Could you check a few things on this drawing? It's one solid part, dimensions in mm from its lowest x, y, z. Give positions to 0.01 mm unless a question says otherwise; leave off trailing zeros. Order: outer loops, then holes, each group sorted by start corner. A loop starts at its lowest first (then second) coordinate and runs counter-clockwise, first axis right, second up. Notation, with made-up numbers: M 20.5,19 L 50.5,19 A17 ccw 50.5,35 Z; hole C -19,-28 d7. An arc over 180 degrees is marked long. Return JSON: item names as keys, results as strings. Group by question number.
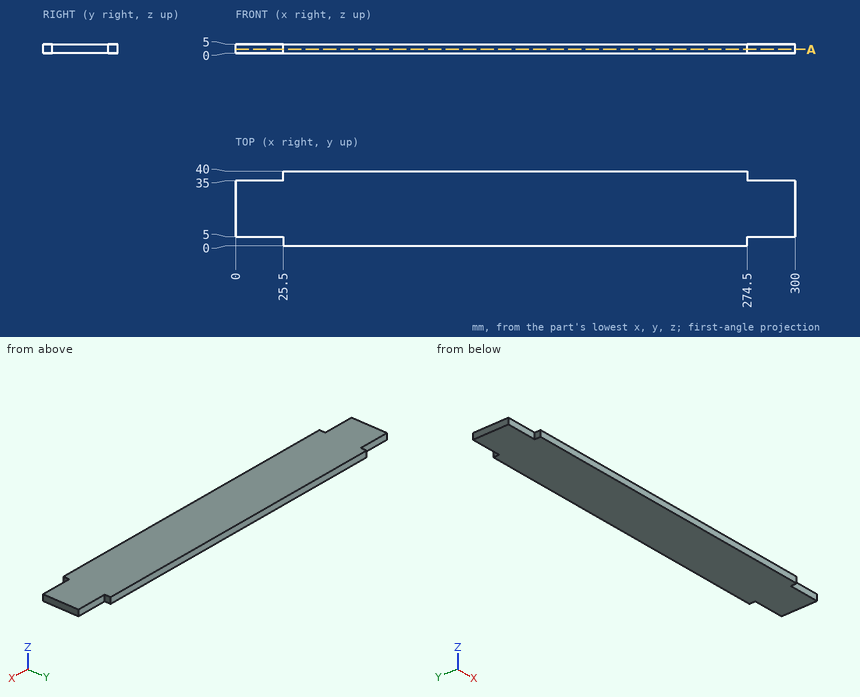
1. Imagine slicing it at A-A, the plane z = 2.1. Please give me the cut outline in (x, y).
2. I need wall thicknesses on L1, parallel to X at y = 3.5, z = 3.1; L2, parallel to Y at x = 284, z = 4.2. Which ranges of each line are inside material? Lowest first, please. Write a range as from..to.
3. For pin 1 (2.5 mm diameter, centred on x = 288, z = 3.5, fed in from +Y); pin 2 (3 mm diameter, centred on y = 32.5, z = 4, fed in from -X); pin 3 (2.5 mm diameter, centred on y = 1.5, z = 2.5, fed in from +X); pin 4 (2.5 mm diameter, centred on x = 292.5, z = 3.5, fed in from -Y), each with a flat end and sliding along its axis, tell me the tip position at first contact or that it passes through.
Values:
{
 "1": {"outline": "M 0,5 L 25.5,5 L 25.5,0 L 274.5,0 L 274.5,5 L 300,5 L 300,35 L 274.5,35 L 274.5,40 L 25.5,40 L 25.5,35 L 0,35 Z"},
 "2": {"L1": "x = 25.5..274.5", "L2": "y = 5..35"},
 "3": {"pin 1": "stops at y = 35", "pin 2": "stops at x = 0", "pin 3": "stops at x = 274.5", "pin 4": "stops at y = 5"}
}
